For this review, take the finished solid that the model builds, in its own axes (mm). A direction names the side the tool comes from. Give positions to 0.01 mm unless a question says otherwise; leave off trailing zeros. Loops run counter-clockwise (first coordinate to the right, second up) from the corner with the lowest first, then second, coordinate; pieces in that order, holes last.
Autodesk Inventor part; units mm, degrees
ref_plane "YZ Plane" through (0, 0, 0) normal (1, 0, 0) x (0, 1, 0)
ref_plane "XZ Plane" through (0, 0, 0) normal (0, 1, 0) x (-1, 0, 0)
ref_plane "XY Plane" through (0, 0, 0) normal (0, 0, 1) x (1, 0, 0)
sketch "Sketch1" plane through (0, 0, 0) normal (0, 0, 1) x (1, 0, 0)
  line L0 (0, 11) -> (-1, 11)
  line L1 (-1, 11) -> (-1, 21)
  line L2 (-1, 21) -> (-2, 21)
  line L3 (-2, 21) -> (-2, 10)
  line L4 (-2, 10) -> (-1.5, 10)
  line L5 (-1.5, 10) -> (-1.5, 0)
  line L6 (-1.5, 0) -> (0, 0)
  line L7 (0, 0) -> (0, 11)
  dimension "d0" = 1
  dimension "d1" = 1.5
  dimension "d3" = 10
  dimension "d5" = 11
  dimension "d9" = 10
  dimension "d12" = 1
revolve "Revolution1" add sketch "Sketch1" angle 360 about axis through (0, 0, 0) along (0, 1, 0)
thread "Thread4"
properties part number "Fitting-2" material "Brass"
Item 1: For L1, parallel to Z at x = 0, y = 16.75; L2, parallel to Y at x = -0.4, z = 1.6, list the stretches that pass through material, from the lowest coordinate up.
Answer:
L1: z = -2 to -1, 1 to 2
L2: y = 10 to 21
Item 2: Tool access review of faces 1 (the flat face through (0, 0, 0)), 2 (the flat face through (0, 11, 0)): name each direction out of +Z, -Z, +X, -X, +Y, -Y from which nothing blocks a thin tool from reaching the whole face with its end or side.
Answer:
face 1: +Z, -Z, +X, -X, -Y
face 2: +Y
Item 3: Clearance check with flat-ended pins moving along their axes: pin 1 Ø1.2 at (x, z) = (0, 0) entering from +Y; pin 2 Ø1.5 at (y, z) = (15.5, -1.5) entering from +X. State where each tip first meets the part, or that it passes through.
Answer:
pin 1: stops at y = 11
pin 2: stops at x = 1.85
Item 4: Take a section at A-A on z = 1.2. Give the boundary of the cut face in (x, y).
Answer:
outline: (-1.6, 10) - (-0.9, 10) - (-0.9, 0) - (0.9, 0) - (0.9, 10) - (1.6, 10) - (1.6, 21) - (-1.6, 21) - close
Item 5: The part is to be moulded in two halves that separate along Z. For faces 3 (the cylindrical face through (0, 16, -1)), 4 (the cylindrical face through (1.5, 4.93, -0.07)), 5 (the flat face through (-1, 21, -1)), say which applies: released by +Z, released by -Z, zero draft, split by the parting line, or undercut.
Answer:
face 3: undercut
face 4: split by the parting line
face 5: zero draft
Item 6: Take a section at D-D on z = 0. Give the boundary of the cut face in (x, y).
Answer:
outline: (-2, 10) - (-1.5, 10) - (-1.5, 0) - (1.5, 0) - (1.5, 10) - (2, 10) - (2, 21) - (1, 21) - (1, 11) - (-1, 11) - (-1, 21) - (-2, 21) - close
Item 7: Take a section at C-C on y = 14.5. Give the boundary of the cut face in (x, z), and give its area (3 significant figures).
Answer:
outline: circle Ø4 at (0, 0); hole circle Ø2 at (0, 0)
area: 9.42 mm2
Item 8: Take a section at B-B on x = 0. Give the boundary of the cut face in (y, z).
Answer:
outline: (0, -1.5) - (10, -1.5) - (10, -2) - (21, -2) - (21, -1) - (11, -1) - (11, 1) - (21, 1) - (21, 2) - (10, 2) - (10, 1.5) - (0, 1.5) - close
